The listing builds one solid part. Answer for the finished solid, in the listing's coordinates (mm). A direction names the side the tool comes from. Coordinates: 2 decimals unless noted, no trailing zeros. Loops run counter-clockwise (first coordinate to the right, second up) from the corner with the lowest first, then second, coordinate; pieces in that order, holes last. Notation, with made-up numbers: (64, -11.5) - (110, -11.5) arc R17 cw to (110, 6.5) - close; hole circle Ø3 at (36, -15.5). An arc over 180 degrees is marked (long way). Return JSON: item names as keys, results as strings. Group by question number.
1. Section C-C (z = 1) is taken. Write down the section's boundary in (x, y), and give its area (3 significant figures).
2. The mould has two halves that part along Z. Classify faces 3 (the face through (0.26, 5.07, 10.23)), 4 (the face through (-15.1, -35, -2)), 5 (the face through (0, 5, -40.492)), 6 (the face through (-23, -35, 5.761)): pulls with the +Z half, pulls with the -Z half, needs draft (parallel to the pull), parting line crosses it, or undercut.
3. Section A-A (x = 0) is taken. Write down the section's boundary in (y, z), and give its area (3 significant figures).
4. Section D-D (y = -41) is taken. Write down the section's boundary in (x, z).
5. Find the intervals of material crossed by line 1 along Z through (x, y) = (-21.5, -18); line 2 along Y through (x, z) = (15, 23.5); line 3 along X through (y, z) = (-23, 0), in increasing order.
6. Which of the six approach directions +Z, -Z, +X, -X, +Y, -Y give full straight-line access (tool end or side, diameter ignored) to faces 1 (the face through (-23, -35, -8.792)), 2 (the face through (31.1, 5, 1))?
7. Each of these flat-tipped pins is pushed along its axis until it touches: P1, Ø3, axis at x = 15, z = 1, coming from the -Y side; P2, Ø4, axis at x = -12.5, y = -50, coming from the -Z side; P3, Ø7.5, axis at y = -24, z = -0.5, coming from the +X side; P4, Ø13, axis at x = -21.5, y = -36, coming from the +Z side. Where does it stop, or does it pass through?
8. Section B-B (z = 14) is taken. Write down the section's boundary in (x, y), and give its area (3 significant figures).
```python
from build123d import *

# Parameters (mm, degrees)
SKETCH1_W           = 62.2
SKETCH1_H           = 80.98413
BOSS_EXTRUDE1_DEPTH = 10
SKETCH2_R           = 5.969
CUT_EXTRUDE1_DEPTH  = 10
SKETCH3_W           = 16
SKETCH3_H           = 14.55264
BOSS_EXTRUDE2_DEPTH = 71.32


with BuildPart() as part:
    # Sketch1 → Boss-Extrude1 (new body)
    with BuildSketch(Plane(origin=(0, 0, 0), x_dir=(1, 0, 0), z_dir=(0, 1, 0))):
        Rectangle(SKETCH1_W, SKETCH1_H)
    extrude(amount=BOSS_EXTRUDE1_DEPTH)

    # Sketch2 → Cut-Extrude1 (cut)
    with BuildSketch(Plane(origin=(0, 10, 0), x_dir=(1, 0, 0), z_dir=(0, 1, 0))):
        with Locations(Location((0, -16.192065, 0), (0, 0, 270))):
            Circle(SKETCH2_R)
    extrude(amount=-CUT_EXTRUDE1_DEPTH, mode=Mode.SUBTRACT)

    # Sketch3 → Boss-Extrude2 (add)
    with BuildSketch(Plane.XZ):
        with Locations((-23.1, -1.515745)):
            Rectangle(SKETCH3_W, SKETCH3_H)
    extrude(amount=BOSS_EXTRUDE2_DEPTH)


solid = part.part
```
The answers:
{
 "1": {"outline": "(-31.1, -71.32) - (-15.1, -71.32) - (-15.1, 0) - (31.1, 0) - (31.1, 10) - (-31.1, 10) - close", "area": "1,760 mm2"},
 "2": {"face 3": "undercut", "face 4": "needs draft", "face 5": "pulls with the -Z half", "face 6": "pulls with the +Z half"},
 "3": {"outline": "(0, -40.49) - (10, -40.49) - (10, 10.22) - (0, 10.22) - close; (0, 22.16) - (10, 22.16) - (10, 40.49) - (0, 40.49) - close", "area": "690 mm2"},
 "4": {"outline": "(-31.1, -8.79) - (-15.1, -8.79) - (-15.1, 5.76) - (-31.1, 5.76) - close"},
 "5": {"line 1": "z = -8.79 to 5.76", "line 2": "y = 0 to 10", "line 3": "x = -31.1 to -15.1"},
 "6": {"face 1": "-Z, +X, -X, -Y", "face 2": "+Z, -Z, +X, +Y, -Y"},
 "7": {"P1": "stops at y = 0", "P2": "passes through", "P3": "stops at x = -15.1", "P4": "stops at z = 5.76"},
 "8": {"outline": "(-31.1, 0) - (-5.55, 0) - (-5.55, 10) - (-31.1, 10) - close; (5.55, 0) - (31.1, 0) - (31.1, 10) - (5.55, 10) - close", "area": "511 mm2"}
}
